The drawing under review shows one solid part. Ordinate dimensions are in mm from its lowest x, y, z. Give positions to 0.01 mm unless a question says otherwise; leave off trailing zeros. Loops run counter-clockwise (first coordinate to the right, second up) from the corner with the lowest first, then second, coordinate; pieces in that order, holes last. Notation, with made-up numbers: M -6.5,22 L -0.5,22 A23 ccw -0.5,48 Z; hole C -22,51.25 d2. An arc over 180 degrees is marked long. Put each result on its own line as item: value. Start each with the question number.
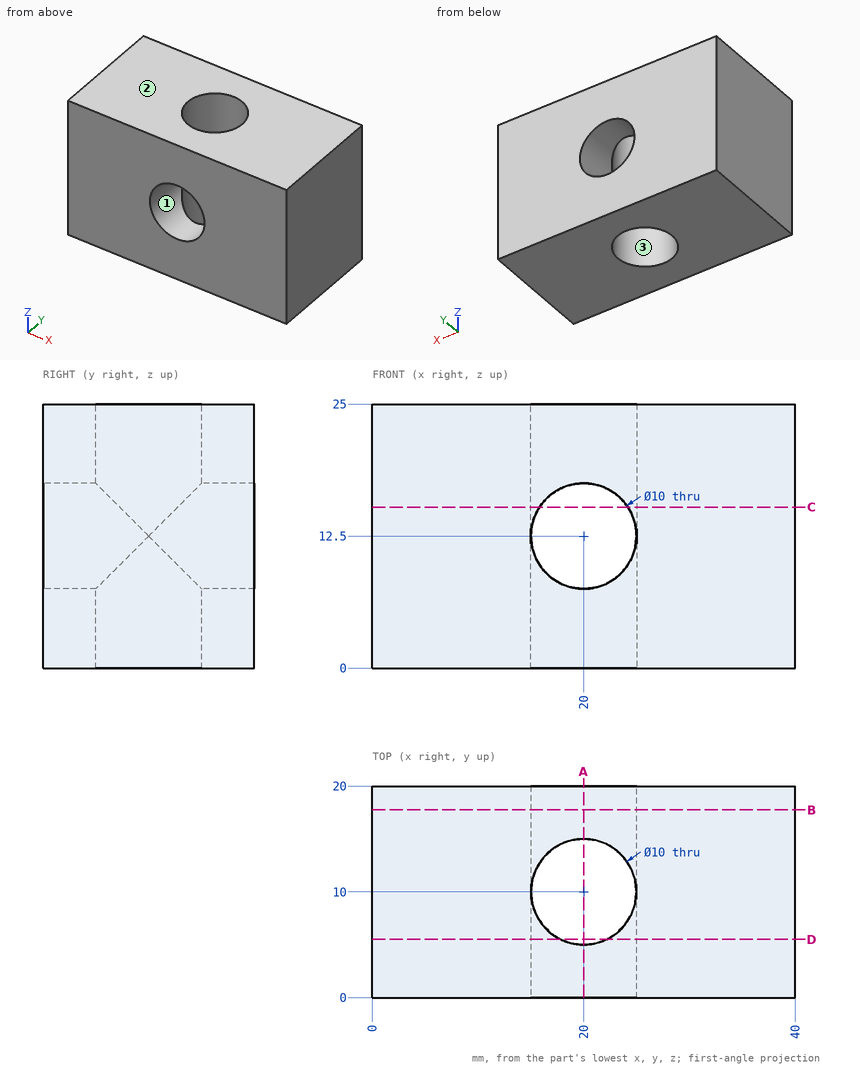
Item 1: Clearance check with flat-ended pins moving along their axes: pin 1 Ø9 at (x, y) = (20, 10) entering from +Z; pin 2 Ø6 at (x, z) = (18.5, 8.5) entering from +Y. State where each tip first meets the part, or that it passes through.
Item 2: Consider section A-A, the plane x = 20. Write out the cut boundary in (y, z).
Item 3: Consider section D-D, the plane y = 5.5. Write out the cut boundary in (x, z), plus the area to 3 significant figures.
Item 4: Draft analysis for pull direction Z (two halves, no side actions). For the marked faces 1, 2 and 3, state which applies: +Z half, -Z half, draft (parallel to the pull), parting line (faces both ways), or undercut.
Item 5: Consider section B-B, the plane y = 17.75. Write out the cut boundary in (x, z), plus the area to 3 significant figures.
Item 6: Consider section C-C, the plane z = 15.25. Write out the cut boundary in (x, y), plus the area to 3 significant figures.
Item 7: To check wall thickness, follow L1, parallel to X at y = 10, z = 8; L2, parallel to Z at x = 20, y = 17.5; L3, parallel to Y at x = 20, z = 6.5. State the ranges of each line that lie inside material, in increasing order. Write a range as [from, to].
Report:
1. pin 1: through
1. pin 2: y = 20
2. outline: M 0,0 L 5,0 L 5,7.5 L 0,7.5 Z; M 0,17.5 L 5,17.5 L 5,25 L 0,25 Z; M 15,0 L 20,0 L 20,7.5 L 15,7.5 Z; M 15,17.5 L 20,17.5 L 20,25 L 15,25 Z
3. outline: M 0,0 L 17.82,0 L 17.82,8 A5 cw 17.82,17 L 17.82,25 L 0,25 Z; M 22.18,0 L 40,0 L 40,25 L 22.18,25 L 22.18,17 A5 cw 22.18,8 Z
3. area: 855 mm²
4. face 1: undercut
4. face 2: +Z half
4. face 3: draft
5. outline: M 0,0 L 40,0 L 40,25 L 0,25 Z; hole C 20,12.5 d10
5. area: 921 mm²
6. outline: M 0,0 L 15.82,0 L 15.82,7.25 A5 cw 15.82,12.75 L 15.82,20 L 0,20 Z; M 24.18,0 L 40,0 L 40,20 L 24.18,20 L 24.18,12.75 A5 cw 24.18,7.25 Z
6. area: 627 mm²
7. L1: [0, 15], [25, 40]
7. L2: [0, 7.5], [17.5, 25]
7. L3: [0, 5], [15, 20]
